Work out the finished part from the listing and answer in its coordinate system (mm). Face numbers are marked on the shaded views. A direction names the side the tool comes from. Coordinates: 2 decimals unless noted, no trailing zeros. Order: outer loops, then holes, each group sorted by start corner. A loop starts at its lowest first (then second) coordinate and runs counter-clockwise, first axis right, second up. Notation, with made-up numbers: (-8.5, 73) - (42.5, 73) arc R26 cw to (42.5, 108) - close; hole circle Ø7 at (1, 20). An arc over 180 degrees is marked (long way). Answer as a JSON object with one key per item and string values. Group by question number.
1) Each of these flat-tipped pins is pushed along its axis until it touches: P1, Ø1, axis at x = 4, z = 1, coming from the +Y side; P2, Ø1.5, axis at y = 4.5, z = 2.5, coming from the -X side. Where does it stop, or does it pass through?
2) The mould has two halves that part along Z. Classify the marked faces 3, 4 and 5: released by +Z, released by -Z, zero draft, split by the parting line, or undercut.
3) Section B-B (z = -1) is taken. Give the vertices of the cut face in (x, y), plus the area to 3 significant figures.
4) Section A-A (x = 1) is taken. Give the vertices of the cut face in (y, z).
5) Section C-C (y = 7.25) is taken. Give the vertices of the cut face in (x, z), plus the area to 3 significant figures.
6) Find the intervals of material crossed by line 1 along Z through (x, y) = (1.25, 5.5); line 2 along X through (y, z) = (7, -1); line 3 along Y through (x, z) = (-0.5, 2.25), in increasing order.
7) A tool of negligible diameter and unlimited length cuts with its end or side. For the marked faces 1 and 2, from which of +Z, -Z, +X, -X, +Y, -Y can it reach the whole face along a straight path? Write none if from no direction.
Autodesk Inventor part; units mm, degrees
ref_plane "YZ Plane" through (0, 0, 0) normal (1, 0, 0) x (0, 1, 0)
ref_plane "XZ Plane" through (0, 0, 0) normal (0, 1, 0) x (-1, 0, 0)
ref_plane "XY Plane" through (0, 0, 0) normal (0, 0, 1) x (1, 0, 0)
sketch "Sketch1" plane through (0, 0, 0) normal (1, 0, 0) x (0, 1, 0)
  point P0 (0, 0)
sketch "Sketch2" plane through (0, 0, 0) normal (0, 1, 0) x (-1, 0, 0)
  line L0 (-6.35, 3.81) -> (6.35, 3.81)
  line L1 (6.35, 3.81) -> (6.35, -3.81)
  line L2 (6.35, -3.81) -> (-6.35, -3.81)
  line L3 (-6.35, -3.81) -> (-6.35, 3.81)
  line L4 (-6.35, 3.81) -> (6.35, -3.81) construction
  line L5 (6.35, 3.81) -> (-6.35, -3.81) construction
  point P0 (0, 0)
  dimension "d0" = 12.7
  dimension "d1" = 7.62
extrude "Extrusion1" add sketch "Sketch2" along normal blind 7.62
sketch "Sketch3" plane through (0, 7.62, 0) normal (0, 1, 0) x (1, 0, 0)
  point P0 (0, 0)
sketch "Sketch4" plane through (-6.35, 0, 3.81) normal (0, 0, 1) x (1, 0, 0)
  line L0 (0, 7.62) -> (12.7, 7.62)
  circle A0 centre (0, 7.62) radius 4.445
  point P0 (6.35, 0)
  dimension "d5" = 8.89
extrude "Extrusion2" cut sketch "Sketch4" against normal blind 12.7
sketch "Sketch5" plane through (0, 7.62, 0) normal (0, 1, 0) x (1, 0, 0)
  point P0 (0, 0)
sketch "Sketch6" plane through (0, 7.62, 0) normal (0, 1, 0) x (1, 0, 0)
  line L0 (6.096, -3.3777) -> (-6.604, -3.3777)
  line L1 (-6.604, -3.3777) -> (-6.604, 3.0508)
  line L2 (-6.604, 3.0508) -> (6.096, 3.0508)
  line L3 (6.096, 3.0508) -> (6.096, -3.3777)
  line L4 (6.35, -3.81) -> (6.35, 3.81)
  point P0 (0, 0)
  dimension "d10" = 12.7
  dimension "d11" = 0.254
extrude "Extrusion3" cut sketch "Sketch6" against normal blind 5.08
properties part number "ScoopBucket"
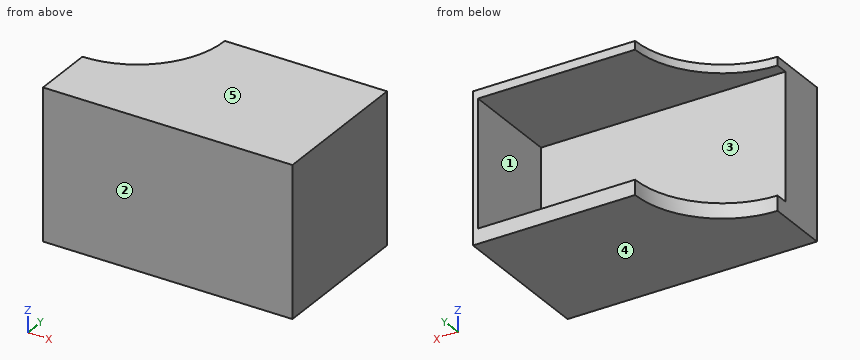
Report:
{
 "1": {"P1": "stops at y = 2.54", "P2": "stops at x = 6.1"},
 "2": {"face 3": "undercut", "face 4": "released by -Z", "face 5": "released by +Z"},
 "3": {"outline": "(-6.35, 0) - (6.35, 0) - (6.35, 7.62) - (6.1, 7.62) - (6.1, 2.54) - (-6.35, 2.54) - close", "area": "33.5 mm²"},
 "4": {"outline": "(0, -3.81) - (7.62, -3.81) - (7.62, -3.05) - (2.54, -3.05) - (2.54, 3.38) - (7.62, 3.38) - (7.62, 3.81) - (0, 3.81) - close"},
 "5": {"outline": "(-1.92, -3.81) - (6.35, -3.81) - (6.35, 3.81) - (-1.92, 3.81) - (-1.92, 3.38) - (6.1, 3.38) - (6.1, -3.05) - (-1.92, -3.05) - close", "area": "11.5 mm²"},
 "6": {"line 1": "z = -3.81 to -3.05, 3.38 to 3.81", "line 2": "x = 6.1 to 6.35", "line 3": "y = 0 to 2.54"},
 "7": {"face 1": "-X, +Y", "face 2": "+Z, -Z, +X, -X, -Y"}
}
